```python
from build123d import *

# Parameters (mm, degrees)
BOSS_EXTRUDE1_DEPTH      = 3
CUT_EXTRUDE21_DEPTH      = 153.533935957
CUT_EXTRUDE21_DEPTH_BACK = 153.533935957
SKETCH34_W               = 3
SKETCH34_H               = 7


with BuildPart() as part:
    # Sketch1 → Boss-Extrude1 (new body)
    with BuildSketch(Plane.XY):
        with BuildLine():
            Line((-65, 90), (-108.301270189, 65))
            ThreePointArc((-108.301270189, 65), (-123.116211843, 0), (-108.301270189, -65))
            Line((-108.301270189, -65), (-65, -90))
            Line((-65, -90), (65, -90))
            Line((65, -90), (108.301270189, -65))
            ThreePointArc((108.301270189, -65), (123.116211843, 0), (108.301270189, 65))
            Line((108.301270189, 65), (65, 90))
            Line((65, 90), (-65, 90))
        make_face()
    extrude(amount=BOSS_EXTRUDE1_DEPTH)

    # Sketch34 → Cut-Extrude21 (cut, two sides: drawn at the far end of the back side and taken through both)
    with BuildSketch(Plane(origin=(0, 0, 0), x_dir=(0, 0, -1), z_dir=(1, 0, 0)).offset(-CUT_EXTRUDE21_DEPTH_BACK)):
        with Locations((-1.5, 86.5)):
            Rectangle(SKETCH34_W, SKETCH34_H)
        with Locations((-1.5, -86.5)):
            Rectangle(SKETCH34_W, SKETCH34_H)
    extrude(amount=CUT_EXTRUDE21_DEPTH + CUT_EXTRUDE21_DEPTH_BACK, mode=Mode.SUBTRACT)


solid = part.part
```
Verification items for the finished model (mm, model axes). Coordinates: 2 decimals unless noted, no trailing zeros. Write each loop counter-clockwise with the first axis right and the second up, starting at its lowest first coordinate (ties: lowest second). Pieces come first, ordered by that corner, then holes. Notation, with made-up numbers: M 63,14 L 85,14 A30 cw 85,42 Z; hole C 23.5,-21 d2. An arc over 180 degrees is marked long. Answer as a JSON object with one key per item and string values. Group by question number.
(1) Cross-section at C-C, the plane y = -72.5. Record the cut outline in (x, z).
(2) Material ranges on line 1 (X direction, y = -14, z = 1.3); line 2 (X direction, y = 44.5, z = 2.7); line 3 (Y direction, x = -84, z = 1.9), recorded low to high.
(3) Gauge pin test, flat end, axial feed: pin 1 (1 mm diameter, centred on x = -86, z = 0.5, fed in from +Y). Record the tip position at first contact, or that the pin passes through.
(4) Cross-section at B-B, the plane x = -87.5. Record the cut outline in (y, z), and give its area (3 significant figures).
(5) Cross-section at A-A, the plane z = 0.95. Record the cut outline in (x, y).
Reply:
{
 "1": {"outline": "M -95.31,0 L 95.31,0 L 95.31,3 L -95.31,3 Z"},
 "2": {"line 1": "-122.46 to 122.46", "line 2": "-116.36 to 116.36", "line 3": "-79.03 to 79.03"},
 "3": {"pin 1": "y = 78.16"},
 "4": {"outline": "M -77.01,0 L 77.01,0 L 77.01,3 L -77.01,3 Z", "area": "462 mm²"},
 "5": {"outline": "M -108.3,-65 L -77.12,-83 L 77.12,-83 L 108.3,-65 A150 ccw 108.3,65 L 77.12,83 L -77.12,83 L -108.3,65 A150 ccw Z"}
}
